Build history of the part. All positions in model axes, mm. A direction names the side the tool comes from. Round coordinates to 2 decimals unless told otherwise and drop trailing zeros. Order: outer loops, then holes, each group sorted by start corner. A loop starts at its lowest first (then second) coordinate and runs counter-clockwise, first axis right, second up. Notation, with made-up numbers: (55.25, 26.5) -> (79.25, 26.5) arc R11 ccw to (79.25, 39.5) -> close; hole circle Ø7 at (76, 61). An arc over 180 degrees is marked (long way). Answer as a JSON object with one key per item and string values.
from build123d import *

# Parameters (mm, degrees)
F0_R       = 25
F1_DEPTH   = 30
F2_R       = 10
F3_DEPTH   = 40
F4_R       = 5
F1_FACE1_R = 25
F5_DEPTH   = 70.001


with BuildPart() as f1:
    # F0 (on Top) → F1 (new body)
    with BuildSketch(Plane.XY):
        Circle(F0_R)
    extrude(amount=F1_DEPTH)

    # F2 (on face) → F3 (join)
    with BuildSketch(Plane.XY.offset(30)):
        Circle(F2_R)
    extrude(amount=F3_DEPTH)

    # F4 (on face) + F1_face1 (on face) → F5 (cut, through all)
    with BuildSketch(Plane.XY.offset(70)):
        Circle(F4_R)
    with BuildSketch(Plane(origin=(0, 0, 0), x_dir=(1, 0, 0), z_dir=(0, 0, -1))):
        Circle(F1_FACE1_R)
    extrude(amount=-F5_DEPTH, dir=(0, 0, 1), mode=Mode.SUBTRACT)


solid = f1.part
1) Pull direction X, two halves, no side cores. Call faces 3 (the face through (-1.08, -4.88, 35.49)), 4 (the face through (-0.3, -5.2, 0)), 5 (the face through (-2.17, -9.76, 49.72)): pulls with the +X half, pulls with the -X half, needs draft (parallel to the pull), parting line crosses it, or undercut.
Checked values:
{"face 3": "undercut", "face 4": "needs draft", "face 5": "parting line crosses it"}
2) Cut at D-D, the plane y = 9. Give the cut face in (x, z), plus the area to 3 significant figures.
Checked values:
{"outline": "(-23.32, 0) -> (23.32, 0) -> (23.32, 30) -> (4.36, 30) -> (4.36, 70) -> (-4.36, 70) -> (-4.36, 30) -> (-23.32, 30) -> close", "area": "1,750 mm²"}
3) Cut at A-A, the plane x = 0. Give the cut face in (y, z), plus the area to 3 significant figures.
Checked values:
{"outline": "(-25, 0) -> (-5, 0) -> (-5, 70) -> (-10, 70) -> (-10, 30) -> (-25, 30) -> close; (5, 0) -> (25, 0) -> (25, 30) -> (10, 30) -> (10, 70) -> (5, 70) -> close", "area": "1,600 mm²"}
4) Which spindle directions (+Z, -Z, +X, -X, +Y, -Y) get a long thin tool onto all of the face, cutting with end or side? Do faces 1 (the face through (-5, -2, 70)), 2 (the face through (0, -11, 30)). Say none if no direction does.
Checked values:
{"face 1": "+Z, +X, -X, +Y, -Y", "face 2": "+Z"}
5) Cut at C-C, the plane z = 10. Give the cut face in (x, y), plus the area to 3 significant figures.
Checked values:
{"outline": "circle Ø50 at (0, 0); hole circle Ø10 at (0, 0)", "area": "1,880 mm²"}
6) Probe L1, parallel to Y at x = 0, z = 53; L2, parallel to Y at x = 0, z = 23; L3, parallel to Z at x = -3.5, y = 15. List the from-to ranges inside material, lowest first. Write a range as from..to.
Checked values:
{"L1": "y = -10..-5, 5..10", "L2": "y = -25..-5, 5..25", "L3": "z = 0..30"}
7) Flat gauge pins, fed straight in: pin 1 Ø3 at (y, z) = (-19.5, 14) entering from -X; pin 2 Ø8 at (x, y) = (15.5, 17.5) entering from +Z; pin 3 Ø4 at (x, z) = (17.5, 26.5) entering from +Y. Where does each tip first touch, or does it go through?
Checked values:
{"pin 1": "stops at x = -17.35", "pin 2": "stops at z = 30", "pin 3": "stops at y = 19.62"}
